Input: dimensioned drawing with shaded views. Units: mm. Origin: part minimum x, y, z. A direction names the side the tool comes from. Coordinates: 2 decimals unless noted, no trailing zeros. Loops run counter-clockwise (first coordinate to the right, second up) from the corner with the lowest first, then second, coordinate; pieces in that order, holes last. Notation, with made-up numbers: (-26.75, -11) -> (-6.75, -11) arc R16 cw to (-6.75, 6) -> close; hole circle Ø10 at (29.25, 82.25). An arc over 180 degrees is marked (long way). Answer as CSV lines item,"result".
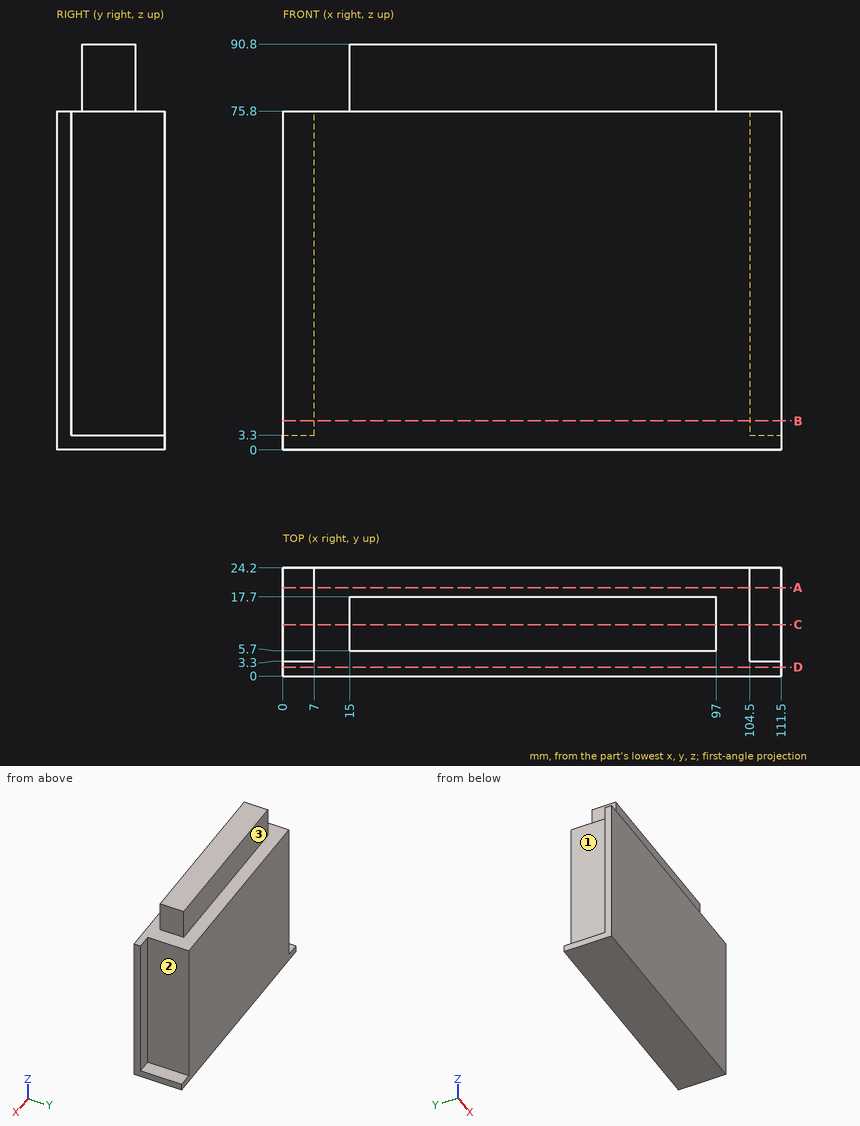
(1) Material intervals for L1, parallel to Z at x = 97.5, y = 7.25; L2, parallel to X at y = 13.5, z = 24.5; L3, parallel to Y at x = 16, z = 85.5, sorted ascending. Write a range as [from, to].
Computed values:
L1,"[0, 75.8]"
L2,"[7, 104.5]"
L3,"[5.7, 17.7]"
(2) Pin query (flat end, axial travel): pin 1 Ø5 at (y, z) = (7, 77.5) entering from -X; pin 2 Ø5.5 at (x, y) = (4.5, 11.5) entering from +Z; pin 3 Ø2 at (x, y) = (88, 2.5) entering from -Z; pin 4 Ø7.5 at (x, z) = (38.5, 85) entering from -Y. Return the tip coordinate at first contact, or that it passes through.
Computed values:
pin 1,"x = 7"
pin 2,"z = 75.8"
pin 3,"z = 0"
pin 4,"y = 5.7"
(3) Cut plane A-A (y = 19.75). Return the cut outline in (x, z).
Computed values:
outline,"(0, 0) -> (111.5, 0) -> (111.5, 3.3) -> (104.5, 3.3) -> (104.5, 75.8) -> (7, 75.8) -> (7, 3.3) -> (0, 3.3) -> close"
(4) Cut plane C-C (y = 11.5). Return the cut outline in (x, z), then the cut area to 3 significant figures.
Computed values:
outline,"(0, 0) -> (111.5, 0) -> (111.5, 3.3) -> (104.5, 3.3) -> (104.5, 75.8) -> (97, 75.8) -> (97, 90.8) -> (15, 90.8) -> (15, 75.8) -> (7, 75.8) -> (7, 3.3) -> (0, 3.3) -> close"
area,"8,670 mm^2"
(5) Cut plane B-B (z = 6.5). Return the cut outline in (x, y), then the cut area to 3 significant figures.
Computed values:
outline,"(0, 0) -> (111.5, 0) -> (111.5, 3.3) -> (104.5, 3.3) -> (104.5, 24.2) -> (7, 24.2) -> (7, 3.3) -> (0, 3.3) -> close"
area,"2,410 mm^2"
(6) Access query for the marked faces 1, 2 and 3. Directions: +Z, -Z, +X, -X, +Y, -Y. A direction counts if a zero-diameter tool reaches every point of the face in a straight line with its end or side. Return the directions, or none.
Computed values:
face 1,"+Z, -X, +Y"
face 2,"+Z, +X, +Y"
face 3,"+Z, +X, -X, +Y"
(7) Cut plane D-D (y = 2). Return the cut outline in (x, z).
Computed values:
outline,"(0, 0) -> (111.5, 0) -> (111.5, 75.8) -> (0, 75.8) -> close"
